Can you work these out from the model? Positions are in its coordinate system, mm. Face numbers are marked on the shaded views. A direction names the side the tool comes from. Round coordinates to 2 decimals unless told otherwise and drop trailing zeros. Loops run counter-clockwise (first coordinate to the right, second up) from the corner with the lowest first, then second, coordinate; pieces in that order, holes last. Notation, with made-up numbers: (38.5, 52.25) -> (79.5, 52.25) arc R19 ccw to (79.5, 87.25) -> close; hole circle Ø4 at (32.25, 21.25). An arc over 180 degrees is marked (long way). Write item = value, one per line.
from build123d import *

# Parameters (mm, degrees)
SKETCH2_R                = 16
BOSS_EXTRUDE1_DEPTH      = 4
BOSS_EXTRUDE2_DEPTH      = 2
BOSS_EXTRUDE2_DEPTH_BACK = 1.5
SKETCH3_R                = 16
SKETCH3_R_2              = 8.25
SKETCH6_W                = 5
SKETCH6_H                = 10
BOSS_EXTRUDE4_DEPTH      = 10
SKETCH7_R                = 1.25
CUT_EXTRUDE2_DEPTH       = 10
SKETCH8_W                = 14
SKETCH8_H                = 12.4
CUT_EXTRUDE3_DEPTH       = 50.94637124


with BuildPart() as part:
    # Sketch2 → Boss-Extrude1 (new, symmetric)
    with BuildSketch(Plane.XY):
        with BuildLine():
            Line((-21, 0), (21, 0))
            Line((21, 0), (21, 23.2))
            ThreePointArc((21, 23.2), (0, 44.2), (-21, 23.2))
            Line((-21, 23.2), (-21, 0))
        make_face()
        with Locations((0, 23.2)):
            Circle(SKETCH2_R, mode=Mode.SUBTRACT)
    extrude(amount=BOSS_EXTRUDE1_DEPTH, both=True)

    # Sketch3 → Boss-Extrude2 (add, two sides: drawn at the far end of the back side and taken through both)
    with BuildSketch(Plane.XY.offset(-BOSS_EXTRUDE2_DEPTH_BACK)):
        with Locations(Location((0, 23.2, 0), (0, 0, 180))):
            Circle(SKETCH3_R)
        with Locations(Location((0, 23.2, 0), (0, 0, 180))):
            Circle(SKETCH3_R_2, mode=Mode.SUBTRACT)
    extrude(amount=BOSS_EXTRUDE2_DEPTH + BOSS_EXTRUDE2_DEPTH_BACK)

    # Sketch6 → Boss-Extrude4 (add)
    with BuildSketch(Plane(origin=(0, 0, -4), x_dir=(-1, 0, 0), z_dir=(0, 0, -1))):
        with Locations((-18.5, 5)):
            Rectangle(SKETCH6_W, SKETCH6_H)
        with Locations((18.5, 5)):
            Rectangle(SKETCH6_W, SKETCH6_H)
    extrude(amount=BOSS_EXTRUDE4_DEPTH)

    # Sketch7 → Cut-Extrude2 (cut)
    with BuildSketch(Plane.XZ):
        with Locations(Location((-18.5, -9, 0), (0, 0, 270))):
            Circle(SKETCH7_R)
        with Locations((18.5, -9)):
            Circle(SKETCH7_R)
        with Locations(Location((-18.5, -1, 0), (0, 0, 270))):
            Circle(SKETCH7_R)
        with Locations((18.5, -1)):
            Circle(SKETCH7_R)
    extrude(amount=-CUT_EXTRUDE2_DEPTH, mode=Mode.SUBTRACT)

    # Sketch8 → Cut-Extrude3 (cut, through all)
    with BuildSketch(Plane(origin=(0, 0, -4), x_dir=(-1, 0, 0), z_dir=(0, 0, -1))):
        Rectangle(SKETCH8_W, SKETCH8_H)
    extrude(amount=-CUT_EXTRUDE3_DEPTH, mode=Mode.SUBTRACT)


solid = part.part
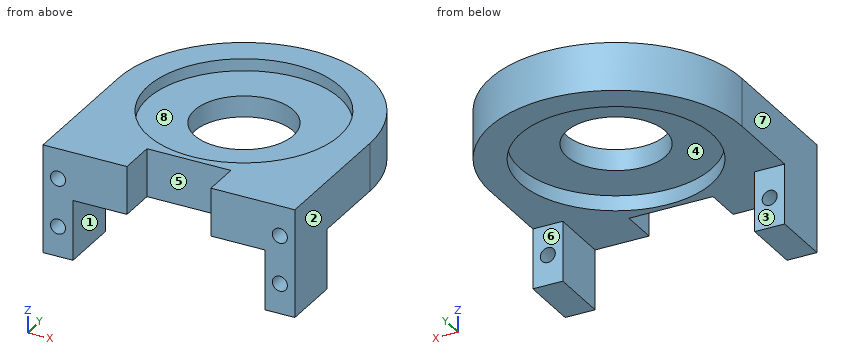
1. We'd pull the mould along Y, two halves only. Please class the marked faces 6, 7 and 8: released by +Y, released by -Y, zero draft, split by the parting line, or undercut.
Entries:
face_6 = released by +Y
face_7 = zero draft
face_8 = undercut
2. I need wall thicknesses on line 1 (Z direction, x = -19, y = 5); line 2 (Y direction, x = 0, z = -3.3); line 3 (X direction, y = 23.2, z = -0.25). Which ranges of each line are inside material? Lowest first, please. Write a range as [from, to].
Entries:
line_1 = [-14, -10.15], [-7.85, -2.15], [0.15, 4]
line_2 = [6.2, 7.2], [39.2, 44.2]
line_3 = [-21, -8.25], [8.25, 21]
3. For the marked faces 1, 2, 3, 4 and 5, which set-ups out of +Z, -Z, +X, -X, +Y, -Y let a thin tool reach every point of the face, with its end or its side?
Entries:
face_1 = -Z, +Y, -Y
face_2 = +Z, -Z, +X, +Y, -Y
face_3 = -Z, +X, -X, +Y
face_4 = -Z
face_5 = +Z, -Z, -Y
4. I'm going to push flat-ended pins straight in: pin 1 (2 mm diameter, centred on x = -18.5, z = -9, fed in from +Y); pin 2 (12.5 mm diameter, centred on x = -2.5, y = 31, fed in from -Z); pin 3 (1.5 mm diameter, centred on x = -10, y = 27.5, fed in from +Z); pin 4 (6 mm diameter, centred on x = 14, z = -8, fed in from +Y). Where does each tip first touch, or does it pass through?
Entries:
pin_1 = through
pin_2 = -1.5
pin_3 = 2
pin_4 = 10
5. Suppose I cut it at C-C, the plane x = 0. List the corners of the cut face in (y, z) for me.
Entries:
outline = (6.2, -4) -> (7.2, -4) -> (7.2, -1.5) -> (14.95, -1.5) -> (14.95, 2) -> (7.2, 2) -> (7.2, 4) -> (6.2, 4) -> close; (31.45, -1.5) -> (39.2, -1.5) -> (39.2, -4) -> (44.2, -4) -> (44.2, 4) -> (39.2, 4) -> (39.2, 2) -> (31.45, 2) -> close
6. Suppose I cut it at A-A, the plane y = 5.5. List the corners of the cut face in (x, z) for me.
Entries:
outline = (-21, -14) -> (-16, -14) -> (-16, -4) -> (-7, -4) -> (-7, 4) -> (-21, 4) -> close; (7, -4) -> (16, -4) -> (16, -14) -> (21, -14) -> (21, 4) -> (7, 4) -> close; hole circle Ø2.5 at (-18.5, -9); hole circle Ø2.5 at (-18.5, -1); hole circle Ø2.5 at (18.5, -9); hole circle Ø2.5 at (18.5, -1)
7. Suppose I cut it at D-D, the plane y = 24.5. List the corners of the cut face in (x, z) for me, and give its area (3 significant figures).
Entries:
outline = (-20.96, -4) -> (-15.95, -4) -> (-15.95, -1.5) -> (-8.15, -1.5) -> (-8.15, 2) -> (-15.95, 2) -> (-15.95, 4) -> (-20.96, 4) -> close; (8.15, -1.5) -> (15.95, -1.5) -> (15.95, -4) -> (20.96, -4) -> (20.96, 4) -> (15.95, 4) -> (15.95, 2) -> (8.15, 2) -> close
area = 135 mm²
8. Suppose I cut it at B-B, the plane z = -11. List the corners of the cut face in (x, y) for me, and give its area (3 significant figures).
Entries:
outline = (-21, 0) -> (-16, 0) -> (-16, 10) -> (-21, 10) -> close; (16, 0) -> (21, 0) -> (21, 10) -> (16, 10) -> close
area = 100 mm²
